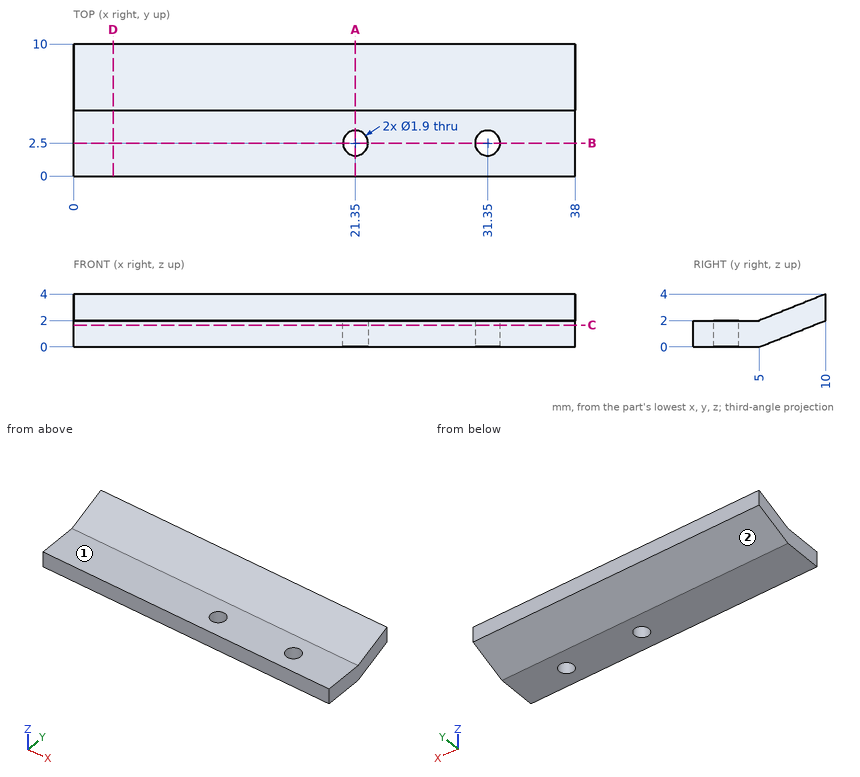
Source: three-view drawing plus pictorial views. Frame: mm from the lowest corner of the part. A direction names the side the tool comes from. Coordinates: 2 decimals unless noted, no trailing zeros. Order: outer loops, then holes, each group sorted by start corner. A loop starts at its lowest first (then second) coordinate and runs counter-clockwise, first axis right, second up. Notation, with made-up numbers: M 3.25,3 L 33.25,3 A14 cw 33.25,29 Z; hole C 87.25,70.5 d8. An arc over 180 degrees is marked long. One line per question, with ' | ' between items. Start each with the question number.
Item 1: Pin query (flat end, axial travel): pin 1 Ø2.5 at (x, y) = (21.35, 2.5) entering from +Z; pin 2 Ø4 at (x, y) = (18.5, 8.5) entering from -Z. Return the tip coordinate at first contact, or that it passes through.
Item 2: Set-up query: the marked faces 1 and 2. Return all of +Z, -Z, +X, -X, +Y, -Y with unobstructed straight access to the full face (end or side cutting, diameter ignored); none if empty.
Item 3: Cut plane C-C, the plane z = 1.65. Return the cut outline in (x, y) (3 decimals), then the cut area to 3 significant figures.
Item 4: Ray query, probe 1 along Z at (x, y) = (10.5, 4.75); probe 2 along Y at (x, z) = (21.35, 1.3); probe 3 along Y at (x, z) = (21.35, 1.55) (3 decimals). Return the intervals inside material, ascending. Write a range as [from, to].
Item 5: Cut plane B-B, the plane y = 2.5. Return the cut outline in (x, z), then the cut area to 3 significant figures.
Item 6: Cut plane A-A, the plane x = 21.35. Return the cut outline in (y, z), then the cut area to 3 significant figures.
Item 7: Cut plane D-D, the plane x = 3. Return the cut outline in (y, z).
A:
1) pin 1: stops at z = 2 | pin 2: stops at z = 0.6
2) face 1: +Z, +X, -X, -Y | face 2: -Z, +X, -X, +Y
3) outline: M 0,0 L 38,0 L 38,9.125 L 0,9.125 Z; hole C 21.35,2.5 d1.9; hole C 31.35,2.5 d1.9 | area: 341 mm2
4) probe 1: z = [0, 2] | probe 2: y = [0, 1.55], [3.45, 8.25] | probe 3: y = [0, 1.55], [3.45, 8.875]
5) outline: M 0,0 L 20.4,0 L 20.4,2 L 0,2 Z; M 22.3,0 L 30.4,0 L 30.4,2 L 22.3,2 Z; M 32.3,0 L 38,0 L 38,2 L 32.3,2 Z | area: 68.4 mm2
6) outline: M 0,0 L 1.55,0 L 1.55,2 L 0,2 Z; M 3.45,0 L 5,0 L 10,2 L 10,4 L 5,2 L 3.45,2 Z | area: 16.2 mm2
7) outline: M 0,0 L 5,0 L 10,2 L 10,4 L 5,2 L 0,2 Z
